Job drawing, mm, ordinate dimensions from the low corner. One solid piece. A direction names the side the tool comes from. Coordinates: 2 decimals unless noted, no trailing zeros. Write each loop counter-clockwise with the first axis right and the second up, starting at its lowest first coordinate (ties: lowest second). Pieces come first, ordered by that corner, then holes. Notation, with made-up numbers: (-19, 88) - (40, 88) arc R7 ccw to (40, 94) - close; hole circle Ø3 at (-39.75, 66). An arc over 180 degrees is marked (long way). Use a Markdown table: item, result.
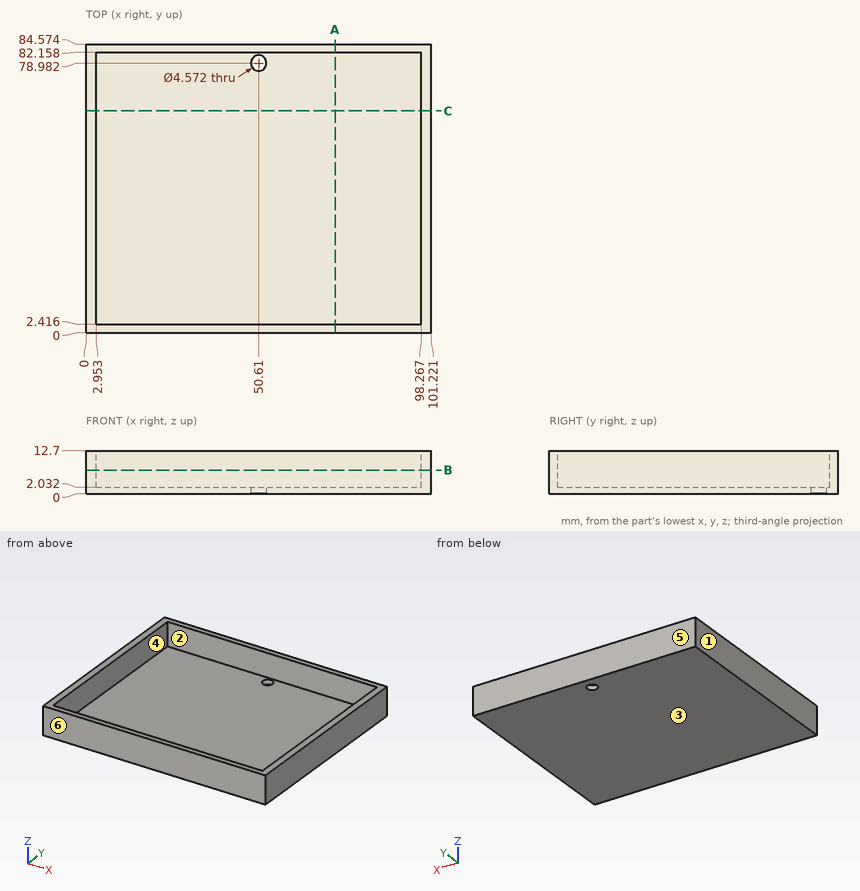
Item 1: Band-saw the part on C-C, the plane y = 65. Give the cut face in (x, z).
From the geometry:
| item | result |
|---|---|
| outline | (0, 0) - (101.22, 0) - (101.22, 12.7) - (98.27, 12.7) - (98.27, 2.03) - (2.95, 2.03) - (2.95, 12.7) - (0, 12.7) - close |
Item 2: Drill centre lines: probe 1 along X at (y, z) = (67.5, 4.75); probe 2 along Y at (x, z) = (25, 6.75) (1 decimal); probe 3 along Z at (x, y) = (54.5, 32). Where is each one in solid material? Low to high.
From the geometry:
| item | result |
|---|---|
| probe 1 | 0 to 2.95, 98.27 to 101.22 |
| probe 2 | 0 to 2.4, 82.2 to 84.6 |
| probe 3 | 0 to 2.03 |
Item 3: Band-saw the part on A-A, the plane x = 73. Give the cut face in (y, z) (1 decimal).
From the geometry:
| item | result |
|---|---|
| outline | (0, 0) - (84.6, 0) - (84.6, 12.7) - (82.2, 12.7) - (82.2, 2) - (2.4, 2) - (2.4, 12.7) - (0, 12.7) - close |
Item 4: Band-saw the part on B-B, the plane z = 7. Give the cut face in (x, y) (1 decimal).
From the geometry:
| item | result |
|---|---|
| outline | (0, 0) - (101.2, 0) - (101.2, 84.6) - (0, 84.6) - close; hole (3, 2.4) - (98.3, 2.4) - (98.3, 82.2) - (3, 82.2) - close |
Item 5: Two-plate mould, pull along Y, no slides. Class the marked faces 3, 4, 5 and 6: pulls with the +Y half, pulls with the -Y half, needs draft (parallel to the pull), parting line crosses it, or undercut.
From the geometry:
| item | result |
|---|---|
| face 3 | needs draft |
| face 4 | undercut |
| face 5 | pulls with the +Y half |
| face 6 | pulls with the -Y half |
Item 6: Which spindle directions (+Z, -Z, +X, -X, +Y, -Y) get a long thin tool onto all of the face, cutting with end or side? Do the marked faces 1 and 2. Say none if no direction does.
From the geometry:
| item | result |
|---|---|
| face 1 | +Z, -Z, -X, +Y, -Y |
| face 2 | +Z |
Item 7: Drop flat-ended pins along their axis: P1, Ø10, axis at x = 29.5, y = 64.5, coming from the +Z side; P2, Ø4, axis at x = 50.61, y = 78.98, coming from the +Z side. Give the stop position or say it passes through.
From the geometry:
| item | result |
|---|---|
| P1 | z = 2.03 |
| P2 | through |
